Geometry check sheet. Reference: the model listing, model coordinates, mm. A direction names the side the tool comes from. Give positions to 0.01 mm unless a question says otherwise; leave off trailing zeros. Write each loop counter-clockwise with the first axis right and the second up, starting at its lowest first coordinate (ties: lowest second). Pieces come first, ordered by that corner, then holes. Notation, with made-up numbers: (73, 84.5) -> (122, 84.5) arc R18 cw to (122, 93.5) -> close; hole circle Ø9 at (-5, 66). An arc over 180 degrees is marked (long way). One line per item, written item: value.
from build123d import *

# Parameters (mm, degrees)
SKETCH1_W           = 58.42
SKETCH1_H           = 10.16
BOSS_EXTRUDE2_DEPTH = 5.08
SKETCH2_W           = 24.504723829
SKETCH2_H           = 7.112
CUT_EXTRUDE1_DEPTH  = 11.938
SKETCH3_W           = 16.975122841
SKETCH3_H           = 18.193068874
CUT_EXTRUDE2_DEPTH  = 11.938
SKETCH4_R           = 2.54
CUT_EXTRUDE3_DEPTH  = 8.382


with BuildPart() as part:
    # Sketch1 → Boss-Extrude2 (new body)
    with BuildSketch(Plane(origin=(0, 0, 0), x_dir=(1, 0, 0), z_dir=(0, 1, 0))):
        with Locations((29.21, -5.08)):
            Rectangle(SKETCH1_W, SKETCH1_H)
    extrude(amount=BOSS_EXTRUDE2_DEPTH)

    # Sketch2 → Cut-Extrude1 (cut)
    with BuildSketch(Plane(origin=(0, 0, 0), x_dir=(1, 0, 0), z_dir=(0, 1, 0))):
        with Locations((12.252361915, -5.08)):
            Rectangle(SKETCH2_W, SKETCH2_H)
    extrude(amount=CUT_EXTRUDE1_DEPTH, mode=Mode.SUBTRACT)

    # Sketch3 → Cut-Extrude2 (cut)
    with BuildSketch(Plane(origin=(0, 0, 0), x_dir=(1, 0, 0), z_dir=(0, 1, 0))):
        with Locations((8.397162409, -3.25308095)):
            Rectangle(SKETCH3_W, SKETCH3_H)
    extrude(amount=CUT_EXTRUDE2_DEPTH, mode=Mode.SUBTRACT)

    # Sketch4 → Cut-Extrude3 (cut)
    with BuildSketch(Plane(origin=(0, 0, 0), x_dir=(1, 0, 0), z_dir=(0, 1, 0))):
        with Locations(Location((41.522723829, -5.27842891, 0), (0, 0, 90))):
            Circle(SKETCH4_R)
    extrude(amount=CUT_EXTRUDE3_DEPTH, mode=Mode.SUBTRACT)


solid = part.part
1) Sectioned sample at C-C on z = 6.25. Record the cut outline in (x, y).
Verdict:
outline: (24.5, 0) -> (39.18, 0) -> (39.18, 5.08) -> (24.5, 5.08) -> close; (43.87, 0) -> (58.42, 0) -> (58.42, 5.08) -> (43.87, 5.08) -> close
2) Depth check by flat-ended pin: pin 1 Ø1 at (y, z) = (3, 5.5) entering from -X. Enter the tip coordinate at first touch or a pass-through.
Verdict:
pin 1: x = 24.5
3) Mould release check, pull along Z, two halves, no side actions. Record for faces 1 (the flat face through (21, 3, 8.636)), 2 (the flat face through (37, 3, 0)), 3 (the flat face through (37, 5.08, 5)): released by +Z, released by -Z, zero draft, split by the parting line, or undercut.
Verdict:
face 1: undercut
face 2: released by -Z
face 3: zero draft
4) Sectioned sample at B-B on y = 0.55. Record the cut outline in (x, z).
Verdict:
outline: (16.88, 0) -> (58.42, 0) -> (58.42, 10.16) -> (16.88, 10.16) -> (16.88, 8.64) -> (24.5, 8.64) -> (24.5, 1.52) -> (16.88, 1.52) -> close; hole circle Ø5.08 at (41.52, 5.28)
5) Tool access check on faces 4 (the flat face through (21, 3, 1.524)), 5 (the flat face through (37, 0, 5)). Record the directions out of +Z, -Z, +X, -X, +Y, -Y that give a thin tool (end or side, any length) a straight path to the whole face; none if there is none.
Verdict:
face 4: -X, +Y, -Y
face 5: +Z, -Z, +X, -X, -Y
6) Sectioned sample at A-A on x = 24. Record the cut outline in (y, z), plus the area to 3 significant figures.
Verdict:
outline: (0, 0) -> (5.08, 0) -> (5.08, 1.52) -> (0, 1.52) -> close; (0, 8.64) -> (5.08, 8.64) -> (5.08, 10.16) -> (0, 10.16) -> close
area: 15.5 mm^2
7) Scan lines: probe 1 along Z at (x, y) = (22, 2.6); probe 2 along X at (y, z) = (0.35, 8.25); probe 3 along X at (y, z) = (3.5, 5.25). Record each from-to range of solid material in increasing order.
Verdict:
probe 1: 0 to 1.52, 8.64 to 10.16
probe 2: 24.5 to 58.42
probe 3: 24.5 to 38.98, 44.06 to 58.42
